Autodesk Inventor part; units mm, degrees
ref_plane "YZ Plane" through (0, 0, 0) normal (1, 0, 0) x (0, 1, 0)
ref_plane "XZ Plane" through (0, 0, 0) normal (0, 1, 0) x (-1, 0, 0)
ref_plane "XY Plane" through (0, 0, 0) normal (0, 0, 1) x (1, 0, 0)
sketch "Sketch1" plane through (0, 0, 0) normal (0, 1, 0) x (-1, 0, 0)
  line L0 (40, 18) -> (-40, 18)
  line L1 (-40, 18) -> (-40, -18)
  line L2 (-40, -18) -> (40, -18)
  line L3 (40, -18) -> (40, 18)
  circle A0 centre (37.5, -15.5) radius 1
  line L4 (37.5, -15.5) -> (-37.5, -15.5) construction
  line L5 (-37.5, -15.5) -> (-37.5, 15.5) construction
  line L6 (-37.5, 15.5) -> (37.5, 15.5) construction
  line L7 (37.5, 15.5) -> (37.5, -15.5) construction
  circle A1 centre (37.5, 15.5) radius 1
  circle A2 centre (-37.5, -15.5) radius 1
  circle A3 centre (-37.5, 15.5) radius 1
  point P0 (0, 0)
  dimension "d0" = 80
  dimension "d1" = 36
  dimension "d2" = 18
  dimension "d3" = 40
  dimension "d4" = 2
  dimension "d5" = 75
  dimension "d6" = 31
  dimension "d7" = 37.5
  dimension "d8" = 15.5
  dimension "d9" = 2
  dimension "d10" = 2
  dimension "d11" = 2
extrude "Extrusion1" add sketch "Sketch1" along normal blind 13.5
properties part number "LCD"
Geometry: final body of the model. Coordinates: model frame, mm. Give positions to 0.01 mm unless a question says otherwise; leave off trailing zeros. Order: outer loops, then holes, each group sorted by start corner. A loop starts at its lowest first (then second) coordinate and runs counter-clockwise, first axis right, second up. Notation, with made-up numbers: (-39.5, 31) - (-17.5, 31) arc R33 cw to (-17.5, 63) - close; hole circle Ø6 at (-6.5, 17). An arc over 180 degrees is marked (long way). Use CSV: the item, a comma, the result in double quotes.
1. Section query A-A (z = -15.5). Output: boundary loops of the cut face in (x, y).
Answers below:
outline,"(-40, 0) - (-38.5, 0) - (-38.5, 13.5) - (-40, 13.5) - close; (-36.5, 0) - (36.5, 0) - (36.5, 13.5) - (-36.5, 13.5) - close; (38.5, 0) - (40, 0) - (40, 13.5) - (38.5, 13.5) - close"
2. Material intervals for line 1 along Z through (x, y) = (37.5, 10), sorted ascending. Write a range as from..to.
Answers below:
line 1,"-18..-16.5, -14.5..14.5, 16.5..18"
3. Contact query for a flat-ended pin moving along its axis: pin 1 (3 mm diameter, centred on x = 19.5, z = 7.5, fed in from -Y). Output: stop coordinate, or through.
Answers below:
pin 1,"y = 0"
4. Section query B-B (x = 37.5). Output: boundary loops of the cut face in (y, z), plus the area to 3 significant figures.
Answers below:
outline,"(0, -18) - (13.5, -18) - (13.5, -16.5) - (0, -16.5) - close; (0, -14.5) - (13.5, -14.5) - (13.5, 14.5) - (0, 14.5) - close; (0, 16.5) - (13.5, 16.5) - (13.5, 18) - (0, 18) - close"
area,"432 mm2"
5. Mould query, pull axis Z, two halves, no side actions, for faces 1 (the face through (-1, 7, 18)), 2 (the face through (-37.96, 6.66, -14.61)), 3 (the face through (1, 13.5, 0)). Classes: +Z half, -Z half, draft (parallel to the pull), parting line (faces both ways), or undercut.
Answers below:
face 1,"+Z half"
face 2,"undercut"
face 3,"draft"
